Input: part model. Units: mm. Frame: model coordinates. Face numbers are marked on the shaded views. A direction names the side the tool comes from. Give positions to 0.01 mm unless a question says otherwise; leave off trailing zeros. Order: outer loops, then holes, each group sorted by start corner. A loop starts at its lowest first (then second) coordinate and runs counter-clockwise, first axis right, second up. Notation, with made-up numbers: (15.5, 75) - (52.5, 75) arc R11 ccw to (52.5, 94) - close; hole circle Ø9 at (52, 75). An arc over 180 degrees is marked (long way). Answer in a Markdown table with one row per item. Add a question column.
from build123d import *

# Parameters (mm, degrees)
F0_W     = 95.377
F0_H     = 25.4
F1_DEPTH = 31.75
F2_T     = -2.778125
F3_W     = 11.1125
F3_H     = 11.1125
F4_DEPTH = 25.401
F5_R     = 2.579688
F6_DEPTH = 95.378


with BuildPart() as f1:
    # F0 (on Top) → F1 (new body, symmetric)
    with BuildSketch(Plane.XY):
        with Locations((47.6885, 12.7)):
            Rectangle(F0_W, F0_H)
    extrude(amount=F1_DEPTH, both=True)

    # F2
    f2_openings = [f1.faces().sort_by_distance(p)[0] for p in [
        (95.377, 12.7, 0),
        (47.6885, 12.7, 31.75),
        (47.6885, 12.7, -31.75),
        (47.6885, 25.4, 0),
    ]]
    offset(amount=F2_T, openings=f2_openings)

    # F3 (on face) → F4 (cut, through all)
    with BuildSketch(Plane.XZ):
        with Locations((76.327, -19.05)):
            Rectangle(F3_W, F3_H)
        with Locations((76.327, 19.05)):
            Rectangle(F3_W, F3_H)
    extrude(amount=-F4_DEPTH, mode=Mode.SUBTRACT)

    # F5 (on face) → F6 (cut, through all)
    with BuildSketch(Plane(origin=(0, 0, 0), x_dir=(0, -1, 0), z_dir=(-1, 0, 0))):
        with Locations((-12.7, 19.05)):
            Circle(F5_R)
        with Locations((-12.7, -19.05)):
            Circle(F5_R)
    extrude(amount=-F6_DEPTH, mode=Mode.SUBTRACT)


solid = f1.part
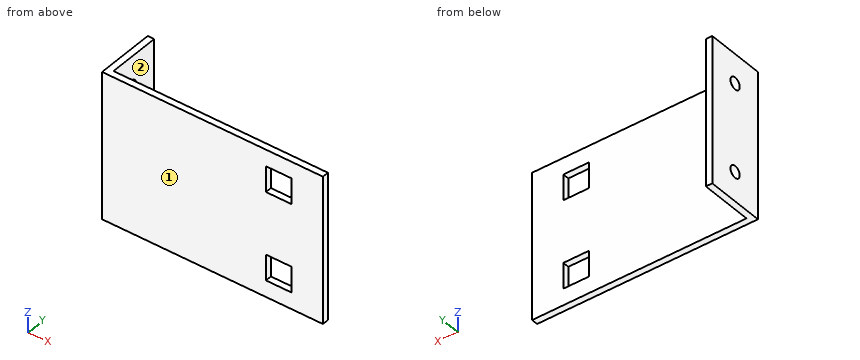
Q1. Contact query for flat-ended pins moving along their axis: P1, Ø6.5, axis at y = 12.7, z = -19.05, coming from the +X side; P2, Ø10, axis at y = 13, z = -14, coming from the -X side; P3, Ø6, axis at x = 56, z = -16.5, coming from the +Y side; P4, Ø12, axis at x = 42, y = 10, coming from the -Z side. Output: stop coordinate, or through.
Q2. Line query: probe 1 along Z at (x, y) = (1.2, 12.7); probe 2 along Y at (x, z) = (1, 19); probe 3 along X at (y, z) = (13.5, 26.5). Output: solid intervals per line, ascending.
Q3. Section C-C, the plane x = 49.5. Return loops of the section in (y, z), then the cut area to 3 significant figures.
Q4. Section D-D, the plane z = 3. Return loops of the section in (x, y).
Q5. Section B-B, the plane y = 12.7. Return loops of the section in (x, z).
Q6. Access query for the marked faces 1 and 2. Directions: +Z, -Z, +X, -X, +Y, -Y. A direction counts if a zero-diameter tool reaches every point of the face in a straight line with its end or side. Return the directions, or none.
Q7. Section A-A, the plane z = 19.05. Return loops of the section in (x, y).
Computed:
| question | item | result |
|---|---|---|
| 1 | P1 | stops at x = 2.78 |
| 1 | P2 | stops at x = 0 |
| 1 | P3 | stops at y = 2.78 |
| 1 | P4 | passes through |
| 2 | probe 1 | z = -31.75 to -21.63, -16.47 to 16.47, 21.63 to 31.75 |
| 2 | probe 2 | y = 0 to 10.12, 15.28 to 25.4 |
| 2 | probe 3 | x = 0 to 2.78 |
| 3 | outline | (0, -31.75) - (2.78, -31.75) - (2.78, 31.75) - (0, 31.75) - close |
| 3 | area | 176 mm^2 |
| 4 | outline | (0, 0) - (95.38, 0) - (95.38, 2.78) - (2.78, 2.78) - (2.78, 25.4) - (0, 25.4) - close |
| 5 | outline | (0, -31.75) - (2.78, -31.75) - (2.78, -21.63) - (0, -21.63) - close; (0, -16.47) - (2.78, -16.47) - (2.78, 16.47) - (0, 16.47) - close; (0, 21.63) - (2.78, 21.63) - (2.78, 31.75) - (0, 31.75) - close |
| 6 | face 1 | +Z, -Z, +X, -X, -Y |
| 6 | face 2 | +Z, -Z, +X, +Y |
| 7 | outline | (0, 0) - (70.77, 0) - (70.77, 2.78) - (2.78, 2.78) - (2.78, 10.12) - (0, 10.12) - close; (0, 15.28) - (2.78, 15.28) - (2.78, 25.4) - (0, 25.4) - close; (81.88, 0) - (95.38, 0) - (95.38, 2.78) - (81.88, 2.78) - close |
